Source: CAD feature listing. Evaluate the final solid. Frame: model axes, mm. A direction names the side the tool comes from. Give positions to 0.01 mm unless a question says otherwise; leave off trailing zeros. Order: outer loops, then holes, each group sorted by start corner. A loop starts at its lowest first (then second) coordinate and runs counter-clockwise, first axis right, second up.
1) Draft query along Z for faces 4 (the face through (-17.4, 2.46, -9.86)), 5 (the face through (35, -5, -7)). Return one class per face: released by +Z, released by -Z, zero draft, split by the parting line, or undercut.
2) Section D-D, the plane z = -39.5. Return loops of the section in (x, y), plus the area to 3 significant figures.
3) Section B-B, the plane x = 0. Return loops of the section in (y, z).
4) Section A-A, the plane y = 2.25. Return loops of the section in (x, z), plus the area to 3 significant figures.
5) Material intervals for line 1 (Y direction, x = -17.5, z = 29.5); line 2 (X direction, y = 1.25, z = -3); line 3 (X direction, y = -2.5, z = -15), sorted ascending.
6) Section C-C, the plane z = 4.5. Return loops of the section in (x, y), plus the area to 3 significant figures.
7) Access query for faces 1 (the face through (1, 5, 22)), 2 (the face through (0, 2, 20)), 3 (the face through (0, 0.5, 46)). Directions: +Z, -Z, +X, -X, +Y, -Y. A direction counts if a zero-diameter tool reaches every point of the face in a straight line with its end or side. Return the directions, or none.
8) First-contact query: P1, Ø1.5, axis at x = 0.5, y = 2, coming from the -Z side; P2, Ø5, axis at y = 1.5, z = -28, coming from the -X side; P3, Ø3, axis at y = -2.5, z = 34, coming from the -X side; P4, Ø11.5, axis at x = -0.5, z = 44.5, coming from the -Y side. Flat tips, straight axial feed; report the tip coordinate or a pass-through.
```python
from build123d import *

# Parameters (mm, degrees)
SKETCH1_R               = 50
BOSS_EXTRUDE1_DEPTH     = 5
BOSS_EXTRUDE2_START     = -5
BOSS_EXTRUDE2_DEPTH     = 5
DRAFT1_ANGLE            = -45
CUT_EXTRUDE2_DEPTH      = 71.887234394
CUT_EXTRUDE2_DEPTH_BACK = 71.887234394
SKETCH1_8_R             = 7.5
CUT_EXTRUDE3_DEPTH      = 71.887234394
CUT_EXTRUDE4_DEPTH      = 0.5
FILLET1_R               = 0.5


with BuildPart() as part:
    # Sketch1 → Boss-Extrude1 (new body)
    with BuildSketch(Plane(origin=(0, 0, 0), x_dir=(1, 0, 0), z_dir=(0, 1, 0))):
        with Locations(Location((0, 0, 0), (0, 0, 270))):
            Circle(SKETCH1_R)
    extrude(amount=BOSS_EXTRUDE1_DEPTH)

    # Sketch1<5> → Boss-Extrude2 (add)
    with BuildSketch(Plane(origin=(0, 0, 0), x_dir=(1, 0, 0), z_dir=(0, 1, 0)).offset(BOSS_EXTRUDE2_START)):
        with BuildLine():
            Line((12.940952255, 48.296291314), (35.355339059, -35.355339059))
            ThreePointArc((35.355339059, -35.355339059), (46.193976626, -19.134171618), (50, 0))
            ThreePointArc((50, 0), (39.667667015, 30.43807145), (12.940952255, 48.296291314))
        make_face()
        with BuildLine():
            ThreePointArc((-12.940952255, 48.296291314), (-48.296291314, 12.940952255), (-35.355339059, -35.355339059))
            Line((-35.355339059, -35.355339059), (-12.940952255, 48.296291314))
        make_face()
    extrude(amount=BOSS_EXTRUDE2_DEPTH)

    # Draft1
    draft1_faces = [part.faces().sort_by_distance(p)[0] for p in [
        (24.148145657, -2.5, -6.470476128),
        (-24.148145657, -2.5, -6.470476128),
    ]]
    draft(draft1_faces, Plane(origin=(0, -5, 0), x_dir=(0, 0, -1), z_dir=(0, -1, 0)), DRAFT1_ANGLE)

    # Sketch1<8> → Cut-Extrude2 (cut, two sides: drawn at the far end of the back side and taken through both)
    with BuildSketch(Plane(origin=(0, 0, 0), x_dir=(1, 0, 0), z_dir=(0, 1, 0)).offset(-CUT_EXTRUDE2_DEPTH_BACK)):
        with Locations(Location((0, -35.355339059, 0), (0, 0, 270))):
            Circle(SKETCH1_8_R)
    extrude(amount=CUT_EXTRUDE2_DEPTH + CUT_EXTRUDE2_DEPTH_BACK, mode=Mode.SUBTRACT)

    # Sketch2 → Cut-Extrude3 (cut, through all)
    with BuildSketch(Plane.XZ):
        Polygon((23.094010768, 0), (11.547005384, 20), (-11.547005384, 20), (-23.094010768, 0), (-11.547005384, -20), (11.547005384, -20), align=None)
    extrude(amount=-CUT_EXTRUDE3_DEPTH, mode=Mode.SUBTRACT)

    # Sketch3 → Cut-Extrude4 (cut)
    with BuildSketch(Plane.XZ):
        with BuildLine():
            ThreePointArc((-7.5, 35.355339059), (0, 42.855339059), (7.5, 35.355339059))
            Line((7.5, 35.355339059), (7.5, 49.434299833))
            ThreePointArc((7.5, 49.434299833), (0, 50), (-7.5, 49.434299833))
            Line((-7.5, 49.434299833), (-7.5, 35.355339059))
        make_face()
    extrude(amount=-CUT_EXTRUDE4_DEPTH, mode=Mode.SUBTRACT)

    # Fillet1
    fillet1_edges = [part.edges().sort_by_distance(p)[0] for p in [
        (0, 0, 27.855339059),
        (-7.5, 0, 42.394819446),
        (7.5, 0, 42.394819446),
    ]]
    fillet(fillet1_edges, radius=FILLET1_R - 0.0001)  # a hair under: the kernel refuses the full size


solid = part.part
```
From the geometry:
1. face 4: undercut
1. face 5: zero draft
2. outline: (-30.66, -5) - (-15.3, -5) - (-20.47, 0) - (20.47, 0) - (15.3, -5) - (30.66, -5) - (30.66, 5) - (-30.66, 5) - close
2. area: 434 mm2
3. outline: (0, -50) - (5, -50) - (5, -20) - (0, -20) - close; (0, 20) - (5, 20) - (5, 27.86) - (0.5, 27.86) arc R0.5 ccw to (0, 27.36) - close; (0.5, 42.86) - (5, 42.86) - (5, 50) - (0.5, 50) - close
4. outline: circle Ø100 at (0, 0); hole (-23.09, 0) - (-11.55, -20) - (11.55, -20) - (23.09, 0) - (11.55, 20) - (-11.55, 20) - close; hole circle Ø15 at (0, 35.36)
4. area: 6,290 mm2
5. line 1: y = 0 to 5
5. line 2: x = -49.91 to -21.36, 21.36 to 49.91
5. line 3: x = -47.7 to -24.45, 24.45 to 47.7
6. outline: (-49.8, -5) - (-27.09, -5) - (-32.26, 0) - (-20.5, 0) - (-20.5, 5) - (-49.8, 5) - close; (20.5, 0) - (32.26, 0) - (27.09, -5) - (49.8, -5) - (49.8, 5) - (20.5, 5) - close
6. area: 494 mm2
7. face 1: +Z, -Z, +X, -X, +Y
7. face 2: +Y, -Y
7. face 3: +Z, -Y
8. P1: stops at z = -50
8. P2: stops at x = -43.01
8. P3: stops at x = -38
8. P4: stops at y = 0.5
